Geometry: final body of the model. Coordinates: model frame, mm. A direction names the side the tool comes from. Coordinates: 2 decimals unless noted, no trailing zeros. Order: outer loops, then holes, each group sorted by start corner. A loop starts at its lowest first (then second) coordinate and runs counter-clockwise, first axis right, second up. Notation, with made-up numbers: M -8.75,71 L 27.25,71 A32 cw 27.25,99 Z; hole C 46.5,-27 d6. An arc over 180 degrees is marked long. Write item = value, one per line. Start each with the question number.
```python
from build123d import *

# Parameters (mm, degrees)
F0_R     = 12.7
F1_DEPTH = 60.325
F3_DEPTH = 19.05
F5_DEPTH = 41.275
F6_R     = 6.35
F7_DEPTH = 57.151
F8_W     = 57.6777060051
F8_H     = 22.3266
F9_DEPTH = 25.4
F10_R    = 7.874
F11_R    = 5.08
F12_R    = 5.08


with BuildPart() as f1:
    # F0 (on Front) → F1 (new body)
    with BuildSketch(Plane.XZ):
        with BuildLine():
            ThreePointArc((22.352, 0), (-15.8052507731, 15.8052507731), (0, -22.352))
            Line((0, -22.352), (194.2084, -22.352))
            Line((194.2084, -22.352), (194.2084, 0))
            Line((194.2084, 0), (150.0886, 0))
            Line((150.0886, 0), (150.0886, 34.798))
            Line((150.0886, 34.798), (131.0386, 34.798))
            ThreePointArc((131.0386, 34.798), (127.4644153616, 16.0823576341), (117.2464, 0))
            Line((117.2464, 0), (85.852, 0))
            Line((85.852, 0), (22.352, 0))
        make_face()
        Circle(F0_R, mode=Mode.SUBTRACT)
    extrude(amount=F1_DEPTH)

    # F2 (on face) → F3 (cut)
    with BuildSketch(Plane.XZ.offset(60.325)):
        Polygon((117.2464, 0), (85.852, 0), (91.8464, -22.352), (117.2464, -22.352), align=None)
    extrude(amount=-F3_DEPTH, mode=Mode.SUBTRACT)

    # F4 (on face) → F5 (cut)
    with BuildSketch(Plane(origin=(0, 0, 0), x_dir=(-1, 0, 0), z_dir=(0, 1, 0))):
        with BuildLine():
            Line((-150.0886, 34.798), (-150.0886, 0))
            Line((-150.0886, 0), (-117.2464, 0))
            ThreePointArc((-117.2464, 0), (-127.4644153616, 16.0823576341), (-131.0386, 34.798))
            Line((-131.0386, 34.798), (-150.0886, 34.798))
        make_face()
    extrude(amount=-F5_DEPTH, mode=Mode.SUBTRACT)

    # F6 (on face) → F7 (cut, through all)
    with BuildSketch(Plane(origin=(0, 0, -22.352), x_dir=(1, 0, 0), z_dir=(0, 0, -1))):
        with Locations((155.3464, 37.973)):
            Circle(F6_R)
    extrude(amount=-F7_DEPTH, mode=Mode.SUBTRACT)

    # F8 (on face) → F9 (cut, symmetric)
    with BuildSketch(Plane.XY):
        with Locations((-6.4868530025, -30.1625)):
            Rectangle(F8_W, F8_H)
    extrude(amount=F9_DEPTH, both=True, mode=Mode.SUBTRACT)

    # F10
    f10_edges = [f1.edges().sort_by_distance(p)[0] for p in [
        (194.2084, -30.1625, 0),
    ]]
    fillet(f10_edges, radius=F10_R)

    # F11
    f11_edges = [f1.edges().sort_by_distance(p)[0] for p in [
        (150.0886, -50.929312, 34.798),
    ]]
    fillet(f11_edges, radius=F11_R)

    # F12
    f12_edges = [f1.edges().sort_by_distance(p)[0] for p in [
        (22.352, -9.4996, 0),
        (22.352, -50.8254, 0),
    ]]
    fillet(f12_edges, radius=F12_R)


solid = f1.part
```
Item 1: Draft query along Z for faces 5 (the flat face through (147, -60.325, 0)), 6 (the cylindrical face through (-16.75, -9.37, 14.8)), 7 (the cylindrical face through (-2.75, -50.69, -12.4)). Return one class per face: pulls with the +Z half, pulls with the -Z half, needs draft (parallel to the pull), parting line crosses it, or undercut.
Item 2: First-contact query: pin 1 (15 mm diameter, centred on x = 0, z = 0, fed in from -Y) (3 decimals); pin 2 (18 mm diameter, centred on x = 106.5, z = -8, fed in from -Y) (3 decimals); pin 3 (16.5 mm diameter, centred on x = 155.35, y = -37.97, fed in from +Z); pin 4 (5.5 mm diameter, centred on y = -50.5, z = 11, fed in from +X). Flat tips, straight axial feed; report the tip coordinate or a pass-through.
Item 3: Section query C-C on x = 136.5. Output: boundary loops of the cut face in (y, z) (3 decimals).
Item 4: Material intervals for probe 1 along Z at (x, y) = (1, -10.5); probe 2 along Z at (x, y) = (0, -7); probe 3 along X at (y, z) = (-45.5, 5), sorted ascending. Write a range as [from, to].
Item 5: Reachability of faces 1 (the cylindrical face through (127.56, -50.67, 16.33)), 2 (the flat face through (150.089, -51, 15)), 3 (the flat face through (22.352, -30, -11)), 4 (the flat face through (88.8, -50.9, -11)) from +Z, -Z, +X, -X, +Y, -Y: full face, straight path, thin tool, end or side. Return the list, or none.
Item 6: Section query D-D on z = 9.5. Output: boundary loops of the cut face in (x, y) (3 decimals), and give its area (3 significant figures).
Item 7: Section query A-A on y = -51. Output: boundary loops of the cut face in (x, z).
Item 8: Section query B-B on z = -4.5. Output: boundary loops of the cut face in (x, y) (3 decimals).
Ans:
q1.face_5 = needs draft
q1.face_6 = parting line crosses it
q1.face_7 = undercut
q2.pin_1 = through
q2.pin_2 = -41.275
q2.pin_3 = 33.97
q2.pin_4 = 150.09
q3.outline = M -60.325,-22.352 L 0,-22.352 L 0,0 L -41.275,0 L -41.275,34.798 L -60.325,34.798 Z
q4.probe_1 = [-22.35, -12.66], [12.66, 22.33]
q4.probe_2 = [-22.35, -12.7], [12.7, 22.35]
q4.probe_3 = [-21.79, -11.67], [11.67, 21.79], [121.38, 150.09]
q5.face_1 = +Z, +Y, -Y
q5.face_2 = +Z, +X, +Y, -Y
q5.face_3 = +Z, -Z, -X
q5.face_4 = +Z, -Y
q6.outline = M -20.233,-60.325 L -8.429,-60.325 L -8.429,-41.326 L -20.233,-41.326 Z; M -20.233,-18.999 L -8.429,-18.999 L -8.429,0 L -20.233,0 Z; M 8.429,-60.325 L 20.233,-60.325 L 20.233,-41.326 L 8.429,-41.326 Z; M 8.429,-18.999 L 20.233,-18.999 L 20.233,0 L 8.429,0 Z; M 124.29,-60.325 L 150.089,-60.325 L 150.089,-41.534 A6.35 cw 149.922,-41.275 L 124.29,-41.275 Z
q6.area = 1,390 mm^2
q7.outline = M 0,-22.35 L 91.85,-22.35 L 85.85,0 L 26.96,0 A5.08 cw 21.97,4.14 A22.35 ccw long Z; M 117.25,-22.35 L 194.21,-22.35 L 194.21,-7.87 A7.87 ccw 186.33,0 L 150.09,0 L 150.09,29.72 A5.08 ccw 145.01,34.8 L 131.04,34.8 A50.8 cw 117.25,0 Z; hole C 0,0 d25.4
q8.outline = M -21.894,-60.325 L -11.876,-60.325 L -11.876,-41.326 L -21.894,-41.326 Z; M -21.894,-18.999 L -11.876,-18.999 L -11.876,0 L -21.894,0 Z; M 11.876,-60.325 L 87.059,-60.325 L 87.059,-41.275 L 117.246,-41.275 L 117.246,-60.325 L 193.449,-60.325 L 193.449,0 L 11.876,0 L 11.876,-18.999 L 22.352,-18.999 L 22.352,-41.326 L 11.876,-41.326 Z; hole C 155.346,-37.973 d12.7
